from build123d import *

# Parameters (mm, degrees)
F0_R     = 31.5235304599
F1_DEPTH = 25
F3_DEPTH = 61
F4_W     = 28.34899351
F4_H     = 30.839510262
F5_DEPTH = 75


with BuildPart() as f1:
    # F0 (on Top) → F1 (new body)
    with BuildSketch(Plane.XY):
        Circle(F0_R)
    extrude(amount=F1_DEPTH)


with BuildPart() as f3:
    # F0 (on Top) → F3 (new body)
    with BuildSketch(Plane.XY):
        Circle(F0_R)
    extrude(amount=F3_DEPTH)

    # F4 (on face) → F5 (cut)
    with BuildSketch(Plane.XY.offset(61)):
        Rectangle(F4_W, F4_H)
    extrude(amount=-F5_DEPTH, mode=Mode.SUBTRACT)


solid = f3.part
Input: part model. Units: mm. Frame: model coordinates. A direction names the side the tool comes from. Give positions to 0.01 mm unless a question says otherwise; leave off trailing zeros. Write each loop counter-clockwise with the first axis right and the second up, starting at its lowest first coordinate (ties: lowest second). Pieces come first, ordered by that corner, then holes. Notation, with made-up numbers: (26.5, 58) -> (44.5, 58) arc R31 cw to (44.5, 83) -> close; hole circle Ø1 at (54, -1.5). An arc over 180 degrees is marked (long way). Use one line per item in the form item = value. Start each with the question number.
1) Section query D-D on y = -21. Return the cut outline in (x, z).
2) Section query C-C on z = 38.5. Return the cut outline in (x, y), then the cut area to 3 significant figures.
3) Pin query (flat end, axial travel): pin 1 (10 mm diameter, centred on x = 5, z = 43, fed in from -Y); pin 2 (9.5 mm diameter, centred on y = 5.5, z = 33.5, fed in from -X); pin 3 (2 mm diameter, centred on x = 10, z = 33, fed in from +Y). Return the tip coordinate at first contact, or that it passes through.
4) Section query B-B on y = 0. Return the cut outline in (x, z).
5) Set-up query: faces 1 (the flat face through (-14.5, 0.4, 0)), 2 (the flat face through (14.174, 0, 31)). Return all of +Z, -Z, +X, -X, +Y, -Y with unobstructed straight access to the full face (end or side cutting, diameter ignored); none if empty.
6) Draft query along X for faces 3 (the flat face through (0, -15.42, 31)), 4 (the cylindrical face through (-4.104, 31.255, 30.073)), 5 (the flat face through (-14.5, 0.4, 61)). Return one class per face: pulls with the +X half, pulls with the -X half, needs draft (parallel to the pull), parting line crosses it, or undercut.
7) Ray query, probe 1 along X at (y, z) = (-14.5, 28.5); probe 2 along X at (y, z) = (3, 31); probe 3 along Y at (x, z) = (-10.5, 21). Return the intervals inside material, ascending. Write a range as from..to.
8) Section query A-A on x = 0. Return the cut outline in (y, z), then the cut area to 3 significant figures.
Outcome:
q1.outline = (-23.51, 0) -> (23.51, 0) -> (23.51, 61) -> (-23.51, 61) -> close
q2.outline = circle Ø63.05 at (0, 0); hole (-14.17, -15.42) -> (14.17, -15.42) -> (14.17, 15.42) -> (-14.17, 15.42) -> close
q2.area = 2,250 mm^2
q3.pin_1 = -31.52
q3.pin_2 = -31.51
q3.pin_3 = 30.21
q4.outline = (-31.52, 0) -> (-14.17, 0) -> (-14.17, 61) -> (-31.52, 61) -> close; (14.17, 0) -> (31.52, 0) -> (31.52, 61) -> (14.17, 61) -> close
q5.face_1 = -Z, +X, -X, +Y, -Y
q5.face_2 = +Z, -Z
q6.face_3 = undercut
q6.face_4 = parting line crosses it
q6.face_5 = needs draft
q7.probe_1 = -27.99..-14.17, 14.17..27.99
q7.probe_2 = -31.38..-14.17, 14.17..31.38
q7.probe_3 = -29.72..-15.42, 15.42..29.72
q8.outline = (-31.52, 0) -> (-15.42, 0) -> (-15.42, 61) -> (-31.52, 61) -> close; (15.42, 0) -> (31.52, 0) -> (31.52, 61) -> (15.42, 61) -> close
q8.area = 1,960 mm^2
